from build123d import *

# Parameters (mm, degrees)
BOSS_EXTRUDE2_DEPTH      = 5
BOSS_EXTRUDE2_DEPTH_BACK = 5
SKETCH1_R                = 3.175


with BuildPart() as part:
    # Sketch1 → Boss-Extrude2 (new, two sides: drawn at the far end of the back side and taken through both)
    with BuildSketch(Plane(origin=(0, 0, 0), x_dir=(1, 0, 0), z_dir=(0, 1, 0)).offset(-BOSS_EXTRUDE2_DEPTH_BACK)):
        with BuildLine():
            ThreePointArc((90, 5), (95, 0), (90, -5))
            Line((90, -5), (-90, -5))
            Line((-90, -5), (-90, 5))
            Line((-90, 5), (90, 5))
        make_face()
        with Locations(Location((90, 0, 0), (0, 0, 270))):
            Circle(SKETCH1_R, mode=Mode.SUBTRACT)
    extrude(amount=BOSS_EXTRUDE2_DEPTH + BOSS_EXTRUDE2_DEPTH_BACK)

    # Sketch8 → Revolve3 (revolve)
    with BuildSketch(Plane(origin=(0, 0, 0), x_dir=(1, 0, 0), z_dir=(0, 1, 0)), mode=Mode.PRIVATE) as revolve3_sk:
        Polygon((-85, -5), (-74.270246445, 5.729753555), (-79.270246445, 5.729753555), (-90, -5), align=None)
    revolve(revolve3_sk.sketch.rotate(Axis((-96.35, 0, -14.166845382), (0, 0, 1)), 180), axis=Axis((-96.35, 0, -14.166845382), (0, 0, 1)))

    # Sketch10 → Cut-Revolve3 (revolve, cut)
    with BuildSketch(Plane(origin=(0, 0, 0), x_dir=(1, 0, 0), z_dir=(0, 1, 0))):
        Polygon((-96.35, 5.729753555), (-79.270246445, 5.729753555), (-90, -5), (-96.35, -5), align=None)
    revolve(axis=Axis((-96.35, 0, -5.729753555), (0, 0, 1)), mode=Mode.SUBTRACT)


solid = part.part
Source: CAD feature listing. Evaluate the final solid. Frame: model axes, mm. Round coordinates to 2 decimals unless told otherwise and drop trailing zeros. Loops run counter-clockwise (first coordinate to the right, second up) from the corner with the lowest first, then second, coordinate; pieces in that order, holes last.
Q1. Ray query, line 1 (Y direction, x = 84, z = 0.25); line 2 (X direction, y = 2.25, z = 0) (3 decimals); line 3 (X direction, y = -2.5, z = -0.25). Return the intervals inside material, ascending.
Q2. Mould query, pull axis Z, two halves, no side actions, for faces 1 (the face through (6, -5, 0)), 2 (the face through (93.15, -0.07, -0.41)), 3 (the face through (-89, 0, 4)). Classes: pulls with the +Z half, pulls with the -Z half, needs draft (parallel to the pull), parting line crosses it, or undercut.
Q3. Section A-A, the plane y = 0. Return loops of the section in (x, z) (3 decimals), plus the area to 3 significant figures.
Q4. Section B-B, the plane x = -96.35. Return loops of the section in (y, z).
Q5. First-contact query: P1, Ø5, axis at x = 13.5, y = -2, coming from the -Z side; P2, Ø6, axis at y = -1.5, z = 1, coming from the -X side; P3, Ø2, axis at y = 12.5, z = -3.5, coming from the +X side. Flat tips, straight axial feed; report the tip coordinate or a pass-through.
Q6. Section C-C, the plane z = 1.5. Return loops of the section in (x, y).
Q7. Section D-D, the plane x = -39. Return loops of the section in (y, z).
Solutions:
1. line 1: y = -5 to 5
1. line 2: x = -112.544 to -107.475, -85.225 to 86.825, 93.175 to 95
1. line 3: x = -112.76 to -107.68, -85.02 to 86.83, 93.17 to 94.99
2. face 1: needs draft
2. face 2: undercut
2. face 3: pulls with the -Z half
3. outline: (-118.43, -5.73) - (-113.43, -5.73) - (-102.7, 5) - (-107.7, 5) - close; (-90, 5) - (-79.27, -5.73) - (-74.27, -5.73) - (-75, -5) - (90, -5) arc R5 ccw to (90, 5) - close; hole circle Ø6.35 at (90, 0)
3. area: 1,810 mm2
4. outline: (-22.08, -5.73) - (-17.08, -5.73) - (-6.35, 5) - (-11.35, 5) - close; (6.35, 5) - (17.08, -5.73) - (22.08, -5.73) - (11.35, 5) - close
5. P1: stops at z = -5
5. P2: stops at x = -114.65
5. P3: stops at x = -79.46
6. outline: (-82.37, -5) - (87.2, -5) - (87.2, 5) - (-82.37, 5) arc R14.85 ccw (long way) to start; (92.8, -5) - (94.77, -5) - (94.77, 5) - (92.8, 5) - close; hole circle Ø19.7 at (-96.35, 0)
7. outline: (-5, -5) - (5, -5) - (5, 5) - (-5, 5) - close
